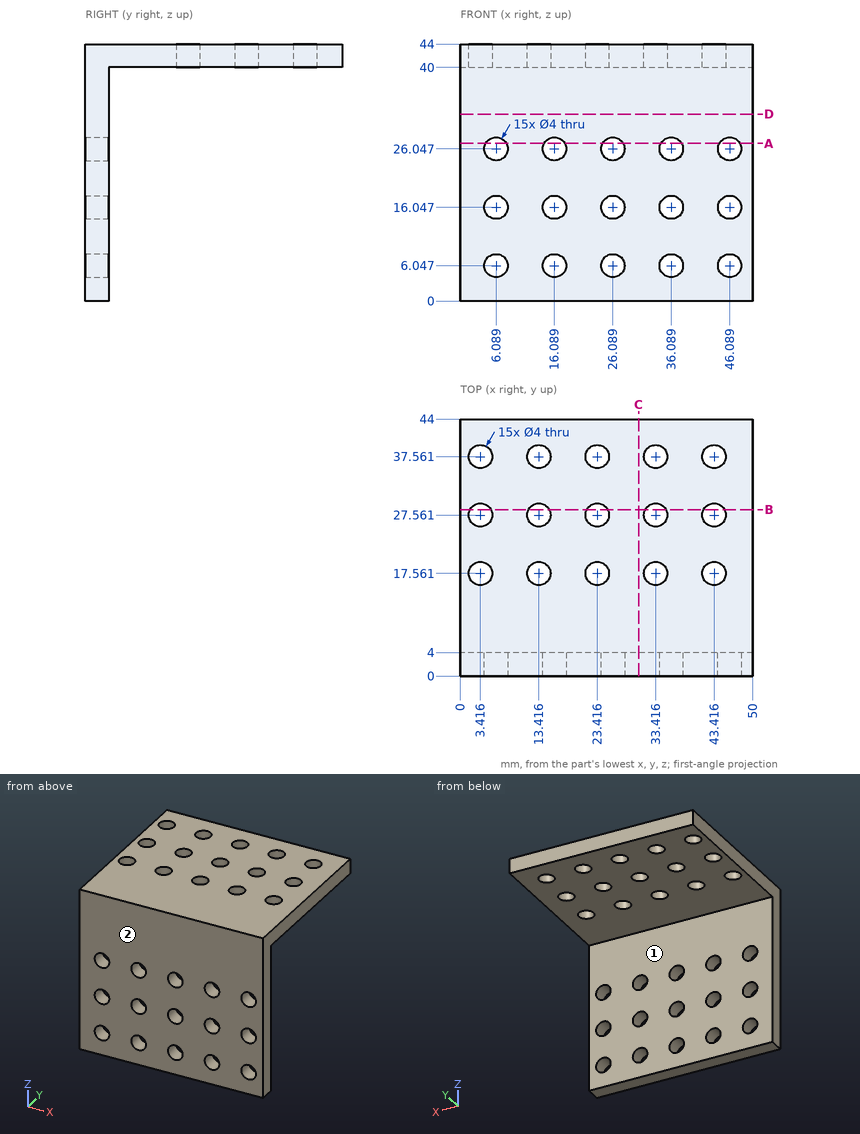
The drawing under review shows one solid part. Ordinate dimensions are in mm from its lowest x, y, z. A direction names the side the tool comes from. Round coordinates to 2 decimals unless told otherwise and drop trailing zeros. Order: outer loops, then holes, each group sorted by start corner. A loop starts at its lowest first (then second) coordinate and runs counter-clockwise, first axis right, second up. Notation, with made-up numbers: (6.25, -39) - (30.25, -39) arc R30 cw to (30.25, -2) - close; hole circle Ø3 at (-40, 53). An arc over 180 degrees is marked (long way). Return JSON: item names as keys, results as strings.
Q1. Consider section D-D on z = 32. Write out the cut boundary in (x, y).
Computed values:
{"outline": "(0, 0) - (50, 0) - (50, 4) - (0, 4) - close"}
Q2. Machinability: for the marked faces 1 and 2, which of the approach directions +Z, -Z, +X, -X, +Y, -Y give a long, thin tool a straight path to every point of the face, cutting with its end or side? Answer none if there is none.
Computed values:
{"face 1": "-Z, +X, -X, +Y", "face 2": "+Z, -Z, +X, -X, -Y"}
Q3. Consider section A-A on z = 27. Write out the cut boundary in (x, y), plus the area to 3 significant figures.
Computed values:
{"outline": "(0, 0) - (4.33, 0) - (4.33, 4) - (0, 4) - close; (7.85, 0) - (14.33, 0) - (14.33, 4) - (7.85, 4) - close; (17.85, 0) - (24.33, 0) - (24.33, 4) - (17.85, 4) - close; (27.85, 0) - (34.33, 0) - (34.33, 4) - (27.85, 4) - close; (37.85, 0) - (44.33, 0) - (44.33, 4) - (37.85, 4) - close; (47.85, 0) - (50, 0) - (50, 4) - (47.85, 4) - close", "area": "130 mm2"}
Q4. For pin 1 Ø6.5 at (x, z) = (36.09, 16.05) entering from +Y; pin 2 Ø6.5 at (x, z) = (6.09, 6.05) entering from -Y; pin 3 Ø6.5 at (x, y) = (23.42, 27.56) entering from -Z, all flat-tipped, find the tip position at first contact; note any pin that passes through.
Computed values:
{"pin 1": "stops at y = 4", "pin 2": "stops at y = 0", "pin 3": "stops at z = 40"}
Q5. Wall thickness on L1, parallel to Y at x = 19, z = 36; L2, parallel to Z at x = 28, y = 33.5: over which ranges is each line inside the solid? List them lowest first. Write a range as [from, to].
Computed values:
{"L1": "y = [0, 4]", "L2": "z = [40, 44]"}
Q6. Consider section B-B on y = 28.5. Write out the cut boundary in (x, z), plus the area to 3 significant figures.
Computed values:
{"outline": "(0, 40) - (1.65, 40) - (1.65, 44) - (0, 44) - close; (5.18, 40) - (11.65, 40) - (11.65, 44) - (5.18, 44) - close; (15.18, 40) - (21.65, 40) - (21.65, 44) - (15.18, 44) - close; (25.18, 40) - (31.65, 40) - (31.65, 44) - (25.18, 44) - close; (35.18, 40) - (41.65, 40) - (41.65, 44) - (35.18, 44) - close; (45.18, 40) - (50, 40) - (50, 44) - (45.18, 44) - close", "area": "129 mm2"}
Q7. Consider section C-C on x = 30.5. Write out the cut boundary in (y, z), plus the area to 3 significant figures.
Computed values:
{"outline": "(0, 0) - (4, 0) - (4, 40) - (44, 40) - (44, 44) - (0, 44) - close", "area": "336 mm2"}
